Read the model definition and answer for the solid it produces. Units are mm, in the model's axes. A direction names the side the tool comes from. Coordinates: 2 decimals unless noted, no trailing zeros. Order: outer loops, then holes, each group sorted by start corner. A loop starts at its lowest first (then second) coordinate and runs counter-clockwise, first axis right, second up. Notation, with made-up numbers: M 75,-37.5 L 111,-37.5 A21 cw 111,-29.5 Z; hole C 69,-28.5 d11. An arc over 180 degrees is marked long. Use a Markdown table: item, result. Add a question column.
1) Find section A-A on y = 14.5. Write down the section's boundary in (x, z).
2) The mould has two halves that part along Y. Classify faces 5 (the face through (2, 18.4, -12)), 6 (the face through (2, 9, -10)), 7 (the face through (1.57, 2.67, -9.59)): released by +Y, released by -Y, zero draft, split by the parting line, or undercut.
3) Find section D-D on y = 50. Write down the section's boundary in (x, z).
4) Find the intervals of material crossed by probe 1 along Y at (x, z) = (1.2, -16.75); probe 2 along Y at (x, z) = (2.8, -15.75); probe 3 along Z at (x, y) = (1.4, 55.31), in increasing order. Write a range as [from, to].
5) Each of these flat-tipped pins is pushed along its axis until it touches: pin 1 Ø1 at (x, y) = (1.5, 9.5) entering from -Z; pin 2 Ø3 at (y, z) = (33.77, -6.59) entering from +X; pin 3 Ø1.6 at (x, y) = (1.5, 53) entering from -Z; pin 4 Ø1.6 at (x, z) = (2.5, -18.5) entering from -Y. Where does it stop, or does it pass through?
6) For faces 1 (the face through (2, 8, 0)), 2 (the face through (2, 49, -20)), 3 (the face through (2, 28.68, -18)), 4 (the face through (2, 15, -21)), determine the directions among +Z, -Z, +X, -X, +Y, -Y from which every point of the face is accessible in a straight line to the end or side of a thin tool.
7) Find section B-B on y = 23.7. Write down the section's boundary in (x, z).
8) Find section C-C on x = 2.5. Count the separate pieces of the cut face and the enclosed holes in it, plus the area to 3 significant figures.
from build123d import *

# Parameters (mm, degrees)
SKETCH1_R                                       = 5
SKETCH1_R_2                                     = 1.6
SKETCH1_R_3                                     = 1.25
BOSS_EXTRUDE1_DEPTH                             = 3.18
CHAMFER1_SIZE                                   = 5
CHAMFER1_SIZE2                                  = 0.881634904
CSK_FOR_M2_FLAT_HEAD_MACHINE_SCREW1_D           = 2.4
CSK_FOR_M2_FLAT_HEAD_MACHINE_SCREW1_DEPTH       = 3.508967257
CSK_FOR_M2_FLAT_HEAD_MACHINE_SCREW1_CSINK_D     = 4.4
CSK_FOR_M2_FLAT_HEAD_MACHINE_SCREW1_CSINK_ANGLE = 90
CSK_FOR_M2_FLAT_HEAD_MACHINE_SCREW1_TIP         = 0.721032743
SKETCH3_R                                       = 5
CUT_EXTRUDE4_DEPTH                              = 64.738438167
FILLET2_R                                       = 3
CHAMFER2_SIZE                                   = 1.8
FILLET4_R                                       = 0.5


with BuildPart() as part:
    # Sketch1 → Boss-Extrude1 (new body)
    with BuildSketch(Plane(origin=(0, 0, 0), x_dir=(0, 0, -1), z_dir=(1, 0, 0))):
        Polygon((0, 0), (0, 16.7), (-2, 18.7), (-2, 28.7), (0, 30.7), (0, 59.81), (20, 59.81), (20, 39.81), (21.8, 39.81), (21.8, 28.68), (13.2, 28.68), (13.2, 18.4), (10.85, 18.4), (10.85, 17), (21, 17), (21, 12), (10, 12), (10, 0), align=None)
        with Locations(Location((5, 23.7, 0), (0, 0, 180))):
            Circle(SKETCH1_R, mode=Mode.SUBTRACT)
        with Locations(Location((5, 55.31, 0), (0, 0, 180))):
            Circle(SKETCH1_R_2, mode=Mode.SUBTRACT)
        with Locations(Location((15, 53.31, 0), (0, 0, 180))):
            Circle(SKETCH1_R_2, mode=Mode.SUBTRACT)
        with Locations(Location((18.5, 14.5, 0), (0, 0, 180))):
            Circle(SKETCH1_R_3, mode=Mode.SUBTRACT)
        with Locations(Location((13.5, 14.5, 0), (0, 0, 180))):
            Circle(SKETCH1_R_3, mode=Mode.SUBTRACT)
    extrude(amount=BOSS_EXTRUDE1_DEPTH)

    # Chamfer1
    chamfer1_edges = [part.edges().sort_by_distance(p)[0] for p in [
        (1.59, 0, -10),
    ]]
    chamfer1_side = [part.faces().sort_by_distance(p)[0] for p in [
        (1.59, 6, -10),
    ]]
    chamfer(chamfer1_edges, length=CHAMFER1_SIZE, length2=CHAMFER1_SIZE2, reference=chamfer1_side[0])

    # CSK for M2 Flat Head Machine Screw1
    with Locations(Plane.ZY):
        with Locations((-4.974936087, 44.914674329), (-15.432559713, 40.744769284), (-6.592504199, 33.773154083)):
            CounterSinkHole(CSK_FOR_M2_FLAT_HEAD_MACHINE_SCREW1_D / 2, CSK_FOR_M2_FLAT_HEAD_MACHINE_SCREW1_CSINK_D / 2, depth=CSK_FOR_M2_FLAT_HEAD_MACHINE_SCREW1_DEPTH, counter_sink_angle=CSK_FOR_M2_FLAT_HEAD_MACHINE_SCREW1_CSINK_ANGLE)
            with Locations((0, 0, -(CSK_FOR_M2_FLAT_HEAD_MACHINE_SCREW1_DEPTH + CSK_FOR_M2_FLAT_HEAD_MACHINE_SCREW1_TIP / 2))):  # 118° drill point
                Cone(0, CSK_FOR_M2_FLAT_HEAD_MACHINE_SCREW1_D / 2, CSK_FOR_M2_FLAT_HEAD_MACHINE_SCREW1_TIP, mode=Mode.SUBTRACT)

    # Sketch3 → Cut-Extrude4 (cut, through all)
    with BuildSketch(Plane.ZY):
        with Locations((-9, 39.810865899)):
            Circle(SKETCH3_R)
    extrude(amount=-CUT_EXTRUDE4_DEPTH, mode=Mode.SUBTRACT)

    # Fillet2
    fillet2_edges = [part.edges().sort_by_distance(p)[0] for p in [
        (1.59, 16.7, 0),
        (1.59, 18.7, 2),
        (1.59, 28.7, 2),
        (1.59, 30.7, 0),
    ]]
    fillet(fillet2_edges, radius=FILLET2_R)

    # Chamfer2
    chamfer2_edges = [part.edges().sort_by_distance(p)[0] for p in [
        (1.59, 59.81, -20),
        (1.59, 59.81, 0),
        (1.59, 39.81, -21.8),
    ]]
    chamfer(chamfer2_edges, length=CHAMFER2_SIZE - 0.0001)  # a hair under: the kernel refuses the full size

    # Fillet4
    fillet4_edges = [part.edges().sort_by_distance(p)[0] for p in [
        (1.59, 38.0101, -21.8),
        (1.59, 58.0101, -20),
        (1.59, 58.0101, 0),
        (1.59, 0, 0),
        (1.59, 18.4, -13.2),
        (1.59, 0, -9.118365096),
    ]]
    fillet(fillet4_edges, radius=FILLET4_R)


solid = part.part
Check result:
| question | item | result |
|---|---|---|
| 1 | outline | M 0,-21 L 3.18,-21 L 3.18,-19.75 L 0,-19.75 Z; M 0,-17.25 L 3.18,-17.25 L 3.18,-14.75 L 0,-14.75 Z; M 0,-12.25 L 3.18,-12.25 L 3.18,0 L 0,0 Z |
| 2 | face 5 | undercut |
| 2 | face 6 | zero draft |
| 2 | face 7 | released by -Y |
| 3 | outline | M 0,-20 L 3.18,-20 L 3.18,0 L 0,0 Z |
| 4 | probe 1 | y = [12, 17], [28.68, 59.81] |
| 4 | probe 2 | y = [12, 17], [28.68, 39.59], [41.9, 51.9], [54.72, 59.81] |
| 4 | probe 3 | z = [-20, -6.6], [-3.4, 0] |
| 5 | pin 1 | stops at z = -10 |
| 5 | pin 2 | stops at x = 3.18 |
| 5 | pin 3 | stops at z = -20 |
| 5 | pin 4 | stops at y = 12 |
| 6 | face 1 | +Z, +X, -X, -Y |
| 6 | face 2 | -Z, +X, -X, +Y |
| 6 | face 3 | -Z, +X, -X |
| 6 | face 4 | -Z, +X, -X, -Y |
| 7 | outline | M 0,-13.2 L 3.18,-13.2 L 3.18,-10 L 0,-10 Z; M 0,0 L 3.18,0 L 3.18,2 L 0,2 Z |
| 8 | separate pieces | 1 |
| 8 | enclosed holes | 9 |
| 8 | area | 839 mm2 |
